Autodesk Inventor part; units mm, degrees
ref_plane "YZ Plane" through (0, 0, 0) normal (1, 0, 0) x (0, 1, 0)
ref_plane "XZ Plane" through (0, 0, 0) normal (0, 1, 0) x (-1, 0, 0)
ref_plane "XY Plane" through (0, 0, 0) normal (0, 0, 1) x (1, 0, 0)
sketch "Sketch1" plane through (0, 0, 0) normal (1, 0, 0) x (0, 1, 0)
  line L0 (-50, 425) -> (50, 425)
  line L1 (50, 425) -> (50, -425)
  line L2 (50, -425) -> (-50, -425)
  line L3 (-50, -425) -> (-50, 425)
  line L4 (-50, 425) -> (50, -425) construction
  line L5 (50, 425) -> (-50, -425) construction
  point P0 (0, 0)
  dimension "d0" = 100
  dimension "d1" = 850
extrude "Extrusion1" add sketch "Sketch1" along normal blind 4
sketch "Sketch2" plane through (4, 0, 0) normal (1, 0, 0) x (0, 0, -1)
  circle A0 centre (-225, -31.7) radius 12.1
  line L0 (-425, -50) -> (425, -50)
  line L1 (-425, 50) -> (-425, -50)
  line L2 (425, 50) -> (-425, 50)
  line L3 (0, 50) -> (0, -50)
  circle A1 centre (225, -31.7) radius 12.1
  point P0 (0, 0)
  dimension "d4" = 18.3
  dimension "d5" = 200
  dimension "d6" = 24.2
  dimension "d9" = 425
extrude "Extrusion2" cut sketch "Sketch2" against normal through all contours A0 | A1
sketch "Sketch3" plane through (4, 0, 0) normal (1, 0, 0) x (0, 0, -1)
  circle A0 centre (120, -42) radius 2.75
  circle A1 centre (120, 42) radius 2.75
  circle A2 centre (0, 37.5) radius 2.75
  circle A3 centre (412.5, 30) radius 2.75
  circle A4 centre (412.5, 0) radius 2.75
  circle A5 centre (412.5, -30) radius 2.75
  circle A6 centre (260, 40.5) radius 2.75
  circle A7 centre (320, 40.5) radius 2.75
  circle A8 centre (145.213, 6.296) radius 10.5
  circle A9 centre (196.913, 6.296) radius 10.5
  circle A10 centre (-145.213, 6.296) radius 10.5
  circle A11 centre (-196.913, 6.296) radius 10.5
  circle A12 centre (-105, -14) radius 10
  circle A13 centre (-79.6, -14) radius 2.75
  circle A14 centre (-130.4, -14) radius 2.75
  circle A15 centre (-264.9997, -22.6996) radius 2.75
  circle A16 centre (-147.163, -33.4172) radius 2.75
  circle A17 centre (264.9997, -22.6996) radius 2.75
  circle A18 centre (174.913, 42.776) radius 2.75
  circle A19 centre (147.163, -33.4172) radius 2.75
  circle A20 centre (130.4, -14) radius 2.75
  circle A21 centre (79.6, -14) radius 2.75
  circle A22 centre (105, 11.4) radius 2.75
  circle A23 centre (105, -39.4) radius 2.75
  circle A24 centre (111.5777, 29.8129) radius 2.75
  circle A25 centre (236.913, 19.219) radius 2.75
  circle A26 centre (-236.913, 19.219) radius 2.75
  circle A27 centre (-174.913, 42.776) radius 2.75
  circle A28 centre (-111.5777, 29.8129) radius 2.75
  circle A29 centre (-105, 11.4) radius 2.75
  circle A30 centre (-105, -39.4) radius 2.75
  circle A31 centre (241, -31.7) radius 2.25
  circle A32 centre (-241, -31.7) radius 2.25
  circle A33 centre (-209, -31.7) radius 2.25
  circle A34 centre (-225, -15.7) radius 2.25
  circle A35 centre (225, -15.7) radius 2.25
  circle A36 centre (209, -31.7) radius 2.25
  circle A37 centre (-225, -31.7) radius 12.3
  circle A38 centre (225, -31.7) radius 12.3
  line L0 (-425, 50) -> (-425, -50)
  line L1 (-425, 50) -> (425, 50)
  line L2 (425, -50) -> (425, 50)
  line L3 (-425, -50) -> (425, -50)
  circle A39 centre (-152.5, 12.5) radius 2.75
  circle A40 centre (152.5, 12.5) radius 2.75
  circle A41 centre (152.5, -12.5) radius 2.75
  circle A42 centre (-152.5, -12.5) radius 2.75
  circle A43 centre (0, -37.5) radius 2.75
  circle A44 centre (320, 40.5) radius 2.75
  circle A45 centre (260, 40.5) radius 2.75
  circle A46 centre (0, 37.5) radius 2.75
  circle A47 centre (120, 42) radius 2.75
  circle A48 centre (380, 40.5) radius 2.75
  circle A49 centre (412.5, 0) radius 2.75
  circle A50 centre (412.5, -30) radius 2.75
  circle A51 centre (-264.9997, -22.6996) radius 2.75
  circle A52 centre (-147.163, -33.4172) radius 2.75
  circle A53 centre (264.9997, -22.6996) radius 2.75
  circle A54 centre (174.913, 42.776) radius 2.75
  circle A55 centre (147.163, -33.4172) radius 2.75
  circle A56 centre (111.5777, 29.8129) radius 2.75
  circle A57 centre (236.913, 19.219) radius 2.75
  circle A58 centre (-236.913, 19.219) radius 2.75
  circle A59 centre (-174.913, 42.776) radius 2.75
  circle A60 centre (-111.5777, 29.8129) radius 2.75
  circle A61 centre (225, -31.7) radius 16.3
  circle A62 centre (-225, -31.7) radius 16.3
  line L4 (-425, -50) -> (-425, 50)
  line L5 (-425, -50) -> (425, -50)
  line L6 (425, 50) -> (425, -50)
  line L7 (-425, 50) -> (425, 50)
  circle A63 centre (-120, 42) radius 2.75
  circle A64 centre (-105, -14) radius 34
  circle A65 centre (75.0667, -42) radius 2.75
  circle A66 centre (105, -14) radius 34
  circle A67 centre (152.5, -12.5) radius 7.5
  circle A68 centre (-152.5, -12.5) radius 7.5
  circle A69 centre (-85.6, 40) radius 2.75
  circle A70 centre (15.6, 40) radius 2.75
  circle A71 centre (364.4, 40) radius 2.75
  circle A72 centre (364.5, -40) radius 2.75
  circle A73 centre (15.6, -40) radius 2.75
  circle A74 centre (-85.6, -40) radius 2.75
  arc A75 (-119.576, -44.7171) -> (-92.3554, -45.5613) centre (-105, -14) ccw
  circle A76 centre (15.6, -40) radius 8.75
  circle A77 centre (-85.6, 40) radius 8.75
  circle A78 centre (15.6, 40) radius 8.75
  circle A79 centre (364.5, -40) radius 8.75
  arc A80 (-92.3554, -45.5613) -> (-78.3455, -35.1077) centre (-85.6, -40) ccw
  circle A81 centre (105, -14) radius 10
  circle A82 centre (0, 0) radius 25
  circle A83 centre (0, 0) radius 25
  arc A84 (119.576, -44.7171) -> (122.4969, -43.1523) centre (120, -42) ccw
  arc A85 (122.4969, -43.1523) -> (119.576, -44.7171) centre (105, -14) ccw
  arc A86 (-78.3455, -35.1077) -> (-122.4969, -43.1523) centre (-105, -14) ccw
  circle A87 centre (412.5, 30) radius 2.75
  circle A88 centre (412.5, 30) radius 2.75
  circle A89 centre (364.4, 40) radius 8.75
  circle A90 centre (364.4, 40) radius 8.75
  circle A91 centre (0, -37.5) radius 7.75
  circle A92 centre (380, 40.5) radius 6.75
  circle A93 centre (-412.5, 0) radius 2.75
  circle A94 centre (-380, 40.5) radius 2.75
  circle A95 centre (-260, 40.5) radius 2.75
  circle A96 centre (-320, 40.5) radius 2.75
  circle A97 centre (-412.5, 30) radius 2.75
  circle A98 centre (-412.5, -30) radius 2.75
  circle A99 centre (-120, -42) radius 2.75
  arc A100 (-122.4969, -43.1523) -> (-119.576, -44.7171) centre (-120, -42) ccw
  circle A101 centre (-412.5, -30) radius 2.75
  circle A102 centre (-412.5, 30) radius 2.75
  circle A103 centre (-320, 40.5) radius 2.75
  circle A104 centre (-260, 40.5) radius 2.75
  circle A105 centre (-380, 40.5) radius 2.75
  circle A106 centre (-412.5, 0) radius 2.75
  circle A107 centre (-120, 42) radius 2.75
  point P0 (0, 0)
  point P1 (72.4969, -43.1523)
  point P2 (69.576, -44.7171)
  point P3 (369.0669, 32.5985)
  point P4 (365.7758, 31.3588)
  point P5 (368.1667, 30)
  point P6 (-105, -14)
  point P7 (-105, -14)
  point P8 (105, -14)
  point P9 (-105, -14)
  point P10 (-105, -14)
extrude "Extrusion3" cut sketch "Sketch3" against normal blind 10 contours A1 | A2 | A4 | A5 | A6 | A7 | A40 A8 | A8 A40 | A39 A10 | A10 A39 | A41 | A42 | A43 picked at (152.3295, 12.2121) picked at (153.6603, 13.4669) picked at (-152.2792, 12.2624) picked at (-153.718, 13.3887)
sketch "Sketch4" plane through (4, 0, 0) normal (1, 0, 0) x (0, 0, -1)
  circle A0 centre (120, 42) radius 2.75
  circle A1 centre (0, 37.5) radius 2.75
  circle A2 centre (-120, 42) radius 2.75
  circle A3 centre (152.5, 12.5) radius 2.75
  circle A4 centre (152.5, -12.5) radius 2.75
  circle A5 centre (-152.5, 12.5) radius 2.75
  circle A6 centre (-152.5, -12.5) radius 2.75
  circle A7 centre (-412.5, 30) radius 2.75
  circle A8 centre (-412.5, 0) radius 2.75
  circle A9 centre (-412.5, -30) radius 2.75
  circle A10 centre (412.5, 30) radius 2.75
  circle A11 centre (412.5, 0) radius 2.75
  circle A12 centre (412.5, -30) radius 2.75
  circle A13 centre (380, 40.5) radius 2.75
  circle A14 centre (320, 40.5) radius 2.75
  circle A15 centre (260, 40.5) radius 2.75
  circle A16 centre (-380, 40.5) radius 2.75
  circle A17 centre (-320, 40.5) radius 2.75
  circle A18 centre (-260, 40.5) radius 2.75
  point P0 (0, 0)
extrude "Extrusion4" cut sketch "Sketch4" against normal through all
properties part number "Bumper Plate" material "Aluminum 6061"
Part model, mm, in its own coordinate system. Coordinates: 2 decimals unless noted, no trailing zeros.
Item 1: Probe line 1 (Y direction, x = 2.7, z = -412.5); line 2 (Y direction, x = 2.65, z = 0); line 3 (Z direction, x = 1.8, y = 12.5). List the from-to ranges inside material, lowest first.
Item 2: Slice it at A-A (x = 0.7). Count the separate pieces of the cut face and the enclosed holes in it, and give its area (3 significant figures).
Item 3: Mould opens along Z. For faces 1 (the face through (2.03, -31.17, 237.09)), 2 (the face through (0, -1, 6)) say: released by +Z, released by -Z, zero draft, split by the parting line, or undercut.
Results found:
1. line 1: y = -50 to -32.75, -27.25 to -2.75, 2.75 to 27.25, 32.75 to 50
1. line 2: y = -50 to -40.25, -34.75 to 34.75, 40.25 to 50
1. line 3: z = -425 to -155.25, -149.75 to 149.75, 155.25 to 425
2. separate pieces: 1
2. enclosed holes: 22
2. area: 83,600 mm2
3. face 1: undercut
3. face 2: zero draft
